Drawing for the job (mm, zero at the part's lowest x, y, z). A direction names the side the tool comes from. Give positions to 0.01 mm unless a question says otherwise; leave off trailing zeros. Order: outer loops, then holes, each group sorted by start corner. A loop starts at its lowest first (then second) coordinate and runs counter-clockwise, first axis right, second up. Notation, with made-up numbers: (59, 57) - (86, 57) arc R12 cw to (86, 74) - close; hole circle Ø5 at (-27, 38.25). An arc over 180 degrees is marked (long way). Use a Markdown table: item, result. Add a question column.
(1) Slice it at A-A (x = 5.08). Write the cut outline in (y, z), then the cut area to 3 significant figures.
(2) Slice it at D-D (x = 15.75). Write the cut outline in (y, z), then the cut area to 3 significant figures.
(3) Mould opens along Z. For the marked faces 6, 7, 8 and 9 say: +Z half, -Z half, draft (parallel to the pull), parting line (faces both ways), or undercut.
(4) Wall check: line 1 (X direction, y = 17.3, z = 97.31); line 2 (Z direction, x = 4, y = 8.5); line 3 (Y direction, x = 16.5, z = 100). Give the ranges that are in metal, low to high.
(5) Flat gauge pins, fed straight in: pin 1 (4 mm diameter, centred on x = 8.5, y = 11.5, fed in from +Z); pin 2 (1.5 mm diameter, centred on y = 3, z = 62.5, fed in from +X); pin 3 (10 mm diameter, centred on x = 9.5, y = 6.5, fed in from -Z); pin 4 (9 mm diameter, centred on x = 8, z = 63.5, fed in from +Y). Where does each tip first touch, or does it go through?
(6) Which spindle directions (+Z, -Z, +X, -X, +Y, -Y) get a long thin tool onto all of the face, cutting with end or side? Do the marked faces 1, 2, 3, 4 and 5. Say none if no direction does.
(7) Slice it at B-B (y = 7). Write the cut outline in (x, z).
(8) Slice it at C-C (z = 10.95). Write the cut outline in (x, y), then the cut area to 3 significant figures.
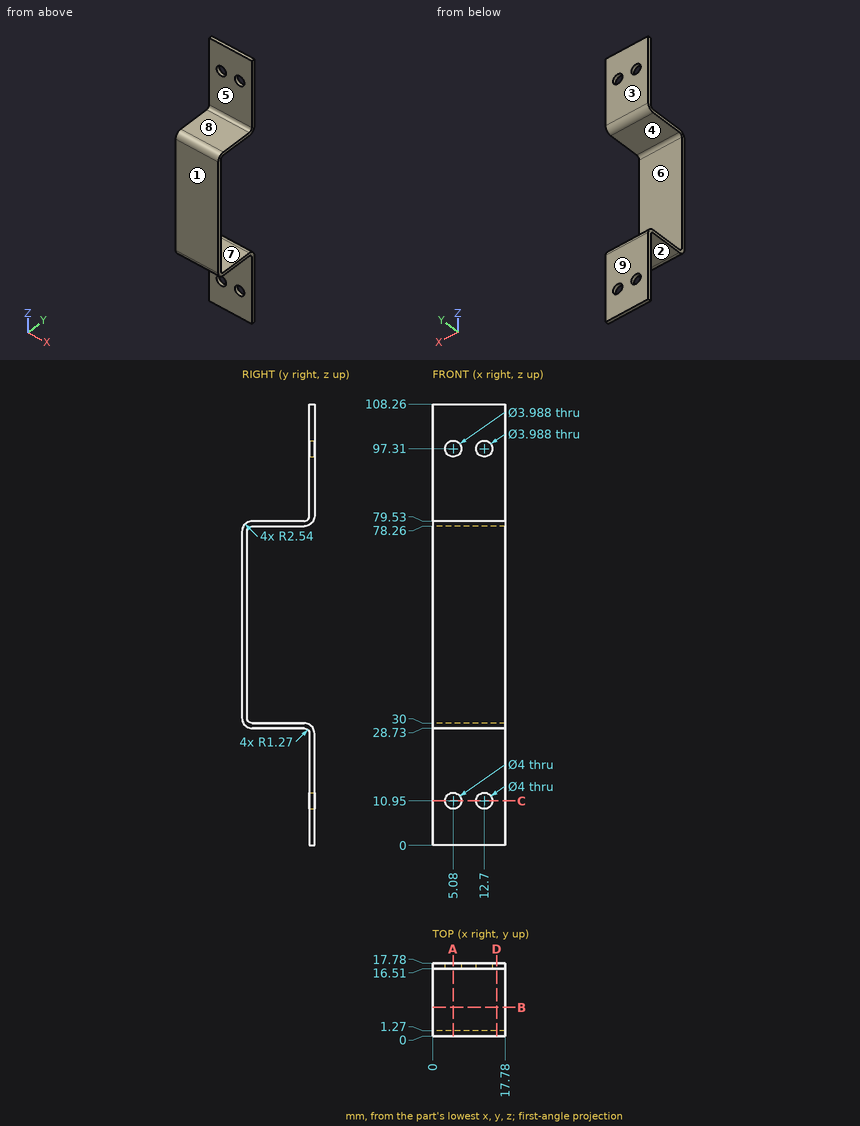
Solution:
| question | item | result |
|---|---|---|
| 1 | outline | (0, 31.27) arc R2.54 ccw to (2.54, 28.73) - (15.24, 28.73) arc R1.27 cw to (16.51, 27.46) - (16.51, 12.95) - (17.78, 12.95) - (17.78, 27.46) arc R2.54 ccw to (15.24, 30) - (2.54, 30) arc R1.27 cw to (1.27, 31.27) - (1.27, 76.99) arc R1.27 cw to (2.54, 78.26) - (15.24, 78.26) arc R2.54 ccw to (17.78, 80.8) - (17.78, 95.32) - (16.51, 95.32) - (16.51, 80.8) arc R1.27 cw to (15.24, 79.53) - (2.54, 79.53) arc R2.54 ccw to (0, 76.99) - close; (16.51, 0) - (17.78, 0) - (17.78, 8.95) - (16.51, 8.95) - close; (16.51, 99.3) - (17.78, 99.3) - (17.78, 108.26) - (16.51, 108.26) - close |
| 1 | area | 165 mm2 |
| 2 | outline | (0, 31.27) arc R2.54 ccw to (2.54, 28.73) - (15.24, 28.73) arc R1.27 cw to (16.51, 27.46) - (16.51, 0) - (17.78, 0) - (17.78, 27.46) arc R2.54 ccw to (15.24, 30) - (2.54, 30) arc R1.27 cw to (1.27, 31.27) - (1.27, 76.99) arc R1.27 cw to (2.54, 78.26) - (15.24, 78.26) arc R2.54 ccw to (17.78, 80.8) - (17.78, 108.26) - (16.51, 108.26) - (16.51, 80.8) arc R1.27 cw to (15.24, 79.53) - (2.54, 79.53) arc R2.54 ccw to (0, 76.99) - close |
| 2 | area | 175 mm2 |
| 3 | face 6 | undercut |
| 3 | face 7 | undercut |
| 3 | face 8 | +Z half |
| 3 | face 9 | draft |
| 4 | line 1 | 0 to 3.09, 7.07 to 10.71, 14.69 to 17.78 |
| 4 | line 2 | 28.73 to 30, 78.26 to 79.53 |
| 4 | line 3 | 16.51 to 17.78 |
| 5 | pin 1 | z = 79.53 |
| 5 | pin 2 | through |
| 5 | pin 3 | z = 28.73 |
| 5 | pin 4 | y = 1.27 |
| 6 | face 1 | +Z, -Z, +X, -X, -Y |
| 6 | face 2 | -Z, +X, -X, -Y |
| 6 | face 3 | +Z, -Z, +X, -X, +Y |
| 6 | face 4 | +X, -X, +Y |
| 6 | face 5 | +Z, +X, -X, -Y |
| 7 | outline | (0, 28.73) - (17.78, 28.73) - (17.78, 30) - (0, 30) - close; (0, 78.26) - (17.78, 78.26) - (17.78, 79.53) - (0, 79.53) - close |
| 8 | outline | (0, 16.51) - (3.08, 16.51) - (3.08, 17.78) - (0, 17.78) - close; (7.08, 16.51) - (10.7, 16.51) - (10.7, 17.78) - (7.08, 17.78) - close; (14.7, 16.51) - (17.78, 16.51) - (17.78, 17.78) - (14.7, 17.78) - close |
| 8 | area | 12.4 mm2 |
